from build123d import *

# Parameters (mm, degrees)
SKETCH1_R                      = 40
SKETCH1_R_2                    = 27.5
BOSS_EXTRUDE1_DEPTH            = 6
SKETCH4_R                      = 40
SKETCH4_R_2                    = 1.65
SKETCH4_R_3                    = 7.5
BOSS_EXTRUDE3_DEPTH            = 6
CBORE_FOR_M2_SHCS1_D           = 2.4
CBORE_FOR_M2_SHCS1_DEPTH       = 12
CBORE_FOR_M2_SHCS1_CBORE_D     = 4.4
CBORE_FOR_M2_SHCS1_CBORE_DEPTH = 8.25


with BuildPart() as part:
    # Sketch1 → Boss-Extrude1 (new body)
    with BuildSketch(Plane(origin=(0, 0, 0), x_dir=(0, 0, -1), z_dir=(1, 0, 0))):
        Circle(SKETCH1_R)
        Circle(SKETCH1_R_2, mode=Mode.SUBTRACT)
    extrude(amount=BOSS_EXTRUDE1_DEPTH)

    # Sketch4 → Boss-Extrude3 (add)
    with BuildSketch(Plane(origin=(6, 0, 8), x_dir=(0, 1, 0), z_dir=(1, 0, 0))):
        with Locations(Location((0, -8, 0), (0, 0, 270))):
            Circle(SKETCH4_R)
        with Locations(Location((-16.22, -8, 0), (0, 0, 270))):
            Circle(SKETCH4_R_2, mode=Mode.SUBTRACT)
        with Locations(Location((16.22, -8, 0), (0, 0, 270))):
            Circle(SKETCH4_R_2, mode=Mode.SUBTRACT)
        with Locations(Location((0, -8, 0), (0, 0, 270))):
            Circle(SKETCH4_R_3, mode=Mode.SUBTRACT)
    extrude(amount=BOSS_EXTRUDE3_DEPTH)

    # CBORE for M2 SHCS1
    with Locations(Plane(origin=(12, 0, 0), x_dir=(0, 0, -1), z_dir=(1, 0, 0))):
        with Locations((0, 0), (-35, 0), (35, 0)):
            CounterBoreHole(CBORE_FOR_M2_SHCS1_D / 2, CBORE_FOR_M2_SHCS1_CBORE_D / 2, CBORE_FOR_M2_SHCS1_CBORE_DEPTH, depth=CBORE_FOR_M2_SHCS1_DEPTH)


solid = part.part
The model under review builds one solid part; all positions refer to its coordinate system, in mm. A direction names the side the tool comes from. Give positions to 0.01 mm unless a question says otherwise; leave off trailing zeros. Order: outer loops, then holes, each group sorted by start corner. A loop starts at its lowest first (then second) coordinate and runs counter-clockwise, first axis right, second up. Notation, with made-up numbers: M -3,-21 L 21,-21 A14 ccw 21,1 Z; hole C 5.25,64 d7. An arc over 180 degrees is marked long. Use one line per item in the form item = value. Start each with the question number.
Item 1: We need section A-A on z = 0. Give the boundary of the cut face in (x, y), plus the area to 3 significant figures.
Item 2: To check wall thickness, follow line 1 along Y through (x, z) = (9.1, 0); line 2 along X through (y, z) = (-7.5, -9); line 3 along Y through (x, z) = (6.75, 35). State the ranges of each line that lie inside material, in increasing order. Write a range as from..to.
Item 3: For faces 4 (the cylindrical face through (1.85, -0.46, -33.89)), 5 (the cylindrical face through (2.958, -26.846, 5.961)), 6 (the flat face through (3.75, -1, -36)), list the 3-axis set-ups (+Z, -Z, +X, -X, +Y, -Y) from which the entire face can be reached by the end or side of a thin tool; tool diameter is ignored.
Item 4: We need section B-B on y = 0. Give the boundary of the cut face in (x, z).
Item 5: The part is to be moulded in two halves that separate along Y. For faces 1 (the flat face through (12, 1, -8)), 2 (the cylindrical face through (5.92, -39.05, 8.67)), 3 (the cylindrical face through (8.96, 14.61, 0.36)), say which applies: pulls with the +Y half, pulls with the -Y half, needs draft (parallel to the pull), parting line crosses it, or undercut.
Item 6: Insertion check: pin 1 Ø1 at (x, z) = (8, -6.5) entering from -Y; pin 2 Ø1.3 at (y, z) = (0.5, 34.5) entering from +X; pin 3 Ø17 at (y, z) = (0, 0) entering from -X. Each pin has a flat end and moves straight along its axis. Give the tip position at first contact, or say it passes through.
Item 7: We need section D-D on z = 35. Give the boundary of the cut face in (x, y), plus the area to 3 significant figures.
Item 8: We need section C-C on y = -16.22. Give the boundary of the cut face in (x, z), plus the area to 3 significant figures.
Completed:
q1.outline = M 0,-40 L 12,-40 L 12,-17.87 L 6,-17.87 L 6,-27.5 L 0,-27.5 Z; M 0,27.5 L 6,27.5 L 6,17.87 L 12,17.87 L 12,40 L 0,40 Z; M 6,-14.57 L 12,-14.57 L 12,-7.5 L 6,-7.5 Z; M 6,7.5 L 12,7.5 L 12,14.57 L 6,14.57 Z
q1.area = 500 mm²
q2.line_1 = -40..-17.87, -14.57..-7.5, 7.5..14.57, 17.87..40
q2.line_2 = 6..12
q2.line_3 = -19.36..-2.2, 2.2..19.36
q3.face_4 = +X, -X
q3.face_5 = -X
q3.face_6 = +X
q4.outline = M 0,-40 L 12,-40 L 12,-37.2 L 3.75,-37.2 L 3.75,-36.2 L 0,-36.2 Z; M 0,-33.8 L 3.75,-33.8 L 3.75,-32.8 L 12,-32.8 L 12,-7.5 L 6,-7.5 L 6,-27.5 L 0,-27.5 Z; M 0,27.5 L 6,27.5 L 6,7.5 L 12,7.5 L 12,32.8 L 3.75,32.8 L 3.75,33.8 L 0,33.8 Z; M 0,36.2 L 3.75,36.2 L 3.75,37.2 L 12,37.2 L 12,40 L 0,40 Z
q5.face_1 = needs draft
q5.face_2 = parting line crosses it
q5.face_3 = undercut
q6.pin_1 = -39.55
q6.pin_2 = 3.75
q6.pin_3 = 6
q7.outline = M 0,-19.36 L 12,-19.36 L 12,-2.2 L 3.75,-2.2 L 3.75,-1.2 L 0,-1.2 Z; M 0,1.2 L 3.75,1.2 L 3.75,2.2 L 12,2.2 L 12,19.36 L 0,19.36 Z
q7.area = 419 mm²
q8.outline = M 0,-36.56 L 12,-36.56 L 12,-1.65 L 6,-1.65 L 6,-22.21 L 0,-22.21 Z; M 0,22.21 L 6,22.21 L 6,1.65 L 12,1.65 L 12,36.56 L 0,36.56 Z
q8.area = 591 mm²
